For this review, take the finished solid that the model builds, in its own axes (mm). Coordinates: 2 decimals unless noted, no trailing zeros. Loops run counter-clockwise (first coordinate to the right, second up) from the corner with the lowest first, then second, coordinate; pieces in that order, holes last. Notation, with made-up numbers: M -5,27.25 L 42,27.25 A19 cw 42,33.25 Z; hole C 41,24.25 d10. An arc over 180 degrees is marked long. Put each result on its own line as item: value.
```python
from build123d import *

# Parameters (mm, degrees)
BOSS_EXTRUDE1_DEPTH = 3
SKETCH2_R           = 11
CUT_EXTRUDE1_DEPTH  = 3
SKETCH3_W           = 35
SKETCH3_H           = 11
CUT_EXTRUDE2_DEPTH  = 3


with BuildPart() as part:
    # Sketch1 → Boss-Extrude1 (new body)
    with BuildSketch(Plane.XY):
        Polygon((450.167740667, -318.916738079), (450.167740667, 1.083261921), (0, 0), (1.167740667, -318.916738079), (36.167740667, -318.916738079), (36.167740667, -338.916738079), (76.167740667, -338.916738079), (76.167740667, -318.916738079), (111.167740667, -318.916738079), (111.167740667, -148.916738079), (114.167740667, -148.916738079), (114.167740667, -318.916738079), (149.167740667, -318.916738079), (149.167740667, -338.916738079), (189.167740667, -338.916738079), (189.167740667, -318.916738079), (224.167740667, -318.916738079), (224.167740667, -148.916738079), (227.167740667, -148.916738079), (227.167740667, -318.916738079), (262.167740667, -318.916738079), (262.167740667, -338.916738079), (302.167740667, -338.916738079), (302.167740667, -318.916738079), (337.167740667, -318.916738079), (337.167740667, -148.916738079), (340.167740667, -148.916738079), (340.167740667, -318.916738079), (375.167740667, -318.916738079), (375.167740667, -338.916738079), (415.167740667, -338.916738079), (415.167740667, -318.916738079), align=None)
    extrude(amount=BOSS_EXTRUDE1_DEPTH)

    # Sketch2 → Cut-Extrude1 (cut)
    with BuildSketch(Plane.XY.offset(3)):
        with Locations((55.20127006, -54.867325568)):
            Circle(SKETCH2_R)
        with Locations((165.20127006, -54.867325568)):
            Circle(SKETCH2_R)
        with Locations((285.167740667, -54.867325568)):
            Circle(SKETCH2_R)
        with Locations((395.167740667, -54.867325568)):
            Circle(SKETCH2_R)
    extrude(amount=-CUT_EXTRUDE1_DEPTH, mode=Mode.SUBTRACT)

    # Sketch3 → Cut-Extrude2 (cut)
    with BuildSketch(Plane.XY.offset(3)):
        with Locations((395.167740667, -303.416738079)):
            Rectangle(SKETCH3_W, SKETCH3_H)
        with Locations((169.167740667, -303.416738079)):
            Rectangle(SKETCH3_W, SKETCH3_H)
        with Locations((282.167740667, -303.416738079)):
            Rectangle(SKETCH3_W, SKETCH3_H)
        with Locations((56.167740667, -303.416738079)):
            Rectangle(SKETCH3_W, SKETCH3_H)
    extrude(amount=-CUT_EXTRUDE2_DEPTH, mode=Mode.SUBTRACT)


solid = part.part
```
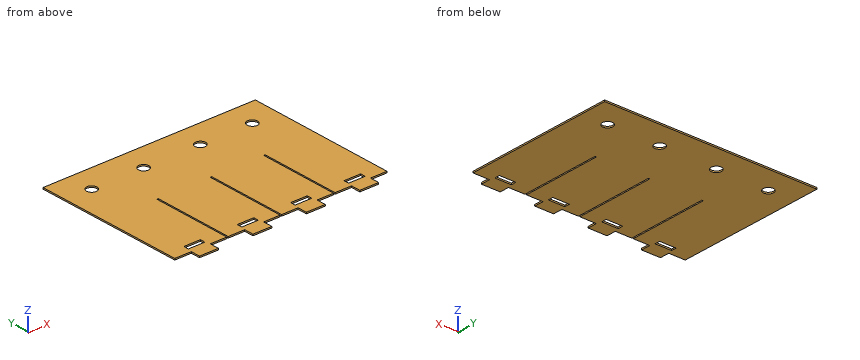
(1) Add section D-D (x = 234.5). Write out the cut boundary in (y, z), plus the area to 3 significant figures.
Determined:
outline: M -318.92,0 L 0.56,0 L 0.56,3 L -318.92,3 Z
area: 958 mm^2
(2) Add section B-B (y = -303.5). State how many separate pieces and enclosed holes the cut face has, plus the area to 3 significant figures.
Determined:
separate pieces: 8
enclosed holes: 0
area: 900 mm^2
(3) Wall thickness on line 1 along X through (y, z) = (-314, 1.1); line 2 along X through (y, z) = (-269, 0.3); line 3 along Y through (x, z) = (280, 0.1): over which ranges is each line inside the solid? List them lowest first. Write a range as [from, to].
Determined:
line 1: x = [1.15, 111.17], [114.17, 224.17], [227.17, 337.17], [340.17, 450.17]
line 2: x = [0.98, 111.17], [114.17, 224.17], [227.17, 337.17], [340.17, 450.17]
line 3: y = [-338.92, -308.92], [-297.92, -64.58], [-45.16, 0.67]
(4) For pin 1 (1.5 mm diameter, centred on y = -230, z = 1.5, fed in from -X); pin 2 (1.5 mm diameter, centred on x = 113, z = 1, fed in from -Y); pin 3 (1 mm diameter, centred on x = 134.5, z = 2.5, fed in from +Y), all flat-tipped, find the tip position at first contact; note any pin that passes through.
Determined:
pin 1: stops at x = 0.84
pin 2: stops at y = -148.92
pin 3: stops at y = 0.32
(5) Add section A-A (y = -253). Write out the cut boundary in (x, z), plus the area to 3 significant figures.
Determined:
outline: M 0.93,0 L 111.17,0 L 111.17,3 L 0.93,3 Z; M 114.17,0 L 224.17,0 L 224.17,3 L 114.17,3 Z; M 227.17,0 L 337.17,0 L 337.17,3 L 227.17,3 Z; M 340.17,0 L 450.17,0 L 450.17,3 L 340.17,3 Z
area: 1,320 mm^2
